from build123d import *

# Parameters (mm, degrees)
SKETCH1_W           = 14
SKETCH1_H           = 20
SKETCH1_R           = 1.25
BOSS_EXTRUDE1_DEPTH = 2
SKETCH2_W           = 10
SKETCH2_H           = 2.5
CUT_EXTRUDE1_DEPTH  = 2


with BuildPart() as part:
    # Sketch1 → Boss-Extrude1 (new body)
    with BuildSketch(Plane.ZY.offset(64.057810508)):
        with Locations((25, -3.601413474)):
            Rectangle(SKETCH1_W, SKETCH1_H)
        with Locations((25, -10.851413474)):
            Circle(SKETCH1_R, mode=Mode.SUBTRACT)
        with Locations((25, 3.648586526)):
            Circle(SKETCH1_R, mode=Mode.SUBTRACT)
    extrude(amount=BOSS_EXTRUDE1_DEPTH)

    # Sketch2 → Cut-Extrude1 (cut)
    with BuildSketch(Plane.ZY.offset(66.057810508)):
        with Locations((25, -2.351413474)):
            Rectangle(SKETCH2_W, SKETCH2_H)
    extrude(amount=-CUT_EXTRUDE1_DEPTH, mode=Mode.SUBTRACT)


solid = part.part
Geometry check sheet. Reference: the model listing, model coordinates, mm. A direction names the side the tool comes from. Round coordinates to 2 decimals unless told otherwise and drop trailing zeros. Loops run counter-clockwise (first coordinate to the right, second up) from the corner with the lowest first, then second, coordinate; pieces in that order, holes last.
Item 1: Access from +Z, -Z, +X, -X, +Y, -Y to the whole of each face (thin tool, end or side, straight path). Record for faces 1 (the flat face through (-65, -3.601, 25)), 2 (the flat face through (-65, -4, 32)).
Item 2: Cross-section at B-B on z = 25. Record the boundary of the cut face in (x, y).
Item 3: Thickness scan on line 1 (Y direction, x = -65.4, z = 25); line 2 (Z direction, x = -65.3, y = -3.5); line 3 (Y direction, x = -64.85, z = 29.5). Record the ranges inside material, lowest first.
Item 4: Cross-section at A-A on z = 28.75. Record the boundary of the cut face in (x, y).
Item 5: Cross-section at C-C on x = -64.9. Record the boundary of the cut face in (y, z).
Item 6: Mould release check, pull along Y, two halves, no side actions. Record for faces 3 (the flat face through (-64.058, -6, 25)), 4 (the flat face through (-65, -2, 30)), 5 (the flat face through (-65, 6.399, 25)): pulls with the +Y half, pulls with the -Y half, needs draft (parallel to the pull), parting line crosses it, or undercut.
Answer sheet:
1. face 1: +X, -X
1. face 2: +Z, +X, -X, +Y, -Y
2. outline: (-66.06, -13.6) - (-64.06, -13.6) - (-64.06, -12.1) - (-66.06, -12.1) - close; (-66.06, -9.6) - (-64.06, -9.6) - (-64.06, -3.6) - (-66.06, -3.6) - close; (-66.06, -1.1) - (-64.06, -1.1) - (-64.06, 2.4) - (-66.06, 2.4) - close; (-66.06, 4.9) - (-64.06, 4.9) - (-64.06, 6.4) - (-66.06, 6.4) - close
3. line 1: y = -13.6 to -12.1, -9.6 to -3.6, -1.1 to 2.4, 4.9 to 6.4
3. line 2: z = 18 to 20, 30 to 32
3. line 3: y = -13.6 to -3.6, -1.1 to 6.4
4. outline: (-66.06, -13.6) - (-64.06, -13.6) - (-64.06, -3.6) - (-66.06, -3.6) - close; (-66.06, -1.1) - (-64.06, -1.1) - (-64.06, 6.4) - (-66.06, 6.4) - close
5. outline: (-13.6, 18) - (6.4, 18) - (6.4, 32) - (-13.6, 32) - close; hole circle Ø2.5 at (-10.85, 25); hole (-3.6, 20) - (-1.1, 20) - (-1.1, 30) - (-3.6, 30) - close; hole circle Ø2.5 at (3.65, 25)
6. face 3: needs draft
6. face 4: undercut
6. face 5: pulls with the +Y half
